The listing builds one solid part. Answer for the finished solid, in the listing's coordinates (mm). Face numbers are marked on the shaded views. A direction names the side the tool comes from. Round coordinates to 2 decimals unless told otherwise and drop trailing zeros. Write each loop counter-clockwise with the first axis right and the second up, starting at its lowest first coordinate (ties: lowest second). Pieces come first, ordered by that corner, then holes. Notation, with made-up numbers: (35, 21.5) - (90, 21.5) arc R14 cw to (90, 44.5) - close; hole circle Ø8 at (-15.5, 87.5). An arc over 180 degrees is marked (long way). Answer in a Markdown table with one row per item.
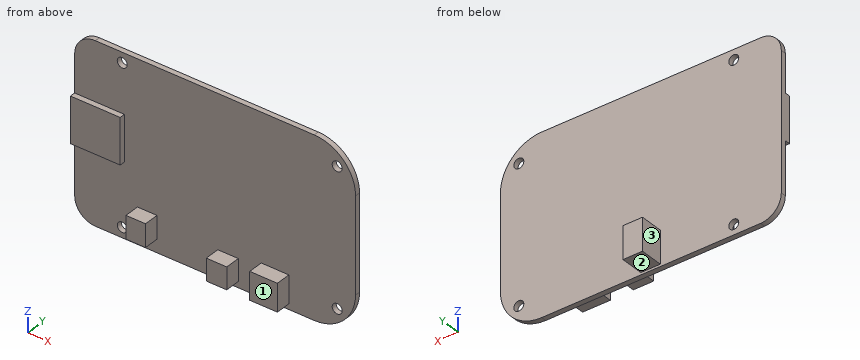
from build123d import *

# Parameters (mm, degrees)
BOSS_EXTRUDE1_DEPTH = 1.6
SKETCH3_R           = 1.53
CUT_EXTRUDE1_DEPTH  = 1.6
SKETCH4_W           = 6
SKETCH4_H           = 10
BOSS_EXTRUDE2_DEPTH = 7.12
SKETCH5_W           = 15.3
SKETCH5_H           = 14
BOSS_EXTRUDE3_DEPTH = 1.7
SKETCH6_W           = 6
SKETCH6_H           = 7
BOSS_EXTRUDE4_DEPTH = 4.6
SKETCH7_W           = 6.3
SKETCH7_H           = 6.75
BOSS_EXTRUDE5_DEPTH = 4.6
SKETCH8_W           = 8.5
SKETCH8_H           = 8.5
BOSS_EXTRUDE6_DEPTH = 4.6


with BuildPart() as part:
    # Sketch1 → Boss-Extrude1 (new body)
    with BuildSketch(Plane(origin=(0, 0, 0), x_dir=(1, 0, 0), z_dir=(0, 1, 0))):
        with BuildLine():
            Line((6.35, 54.61), (73.66, 54.61))
            ThreePointArc((73.66, 54.61), (82.640256121, 50.890256121), (86.36, 41.91))
            Line((86.36, 41.91), (86.36, 12.7))
            ThreePointArc((86.36, 12.7), (82.640256121, 3.719743879), (73.66, 0))
            Line((73.66, 0), (6.35, 0))
            ThreePointArc((6.35, 0), (1.859871939, 1.859871939), (0, 6.35))
            Line((0, 6.35), (0, 48.26))
            ThreePointArc((0, 48.26), (1.859871939, 52.750128061), (6.35, 54.61))
        make_face()
    extrude(amount=BOSS_EXTRUDE1_DEPTH)

    # Sketch3 → Cut-Extrude1 (cut)
    with BuildSketch(Plane(origin=(0, 1.6, 0), x_dir=(1, 0, 0), z_dir=(0, 1, 0))):
        with Locations(Location((80.71, 6.35, 0), (0, 0, 270))):
            Circle(SKETCH3_R)
        with Locations(Location((14.61, 3.11, 0), (0, 0, 270))):
            Circle(SKETCH3_R)
        with Locations(Location((14.61, 51.5, 0), (0, 0, 270))):
            Circle(SKETCH3_R)
        with Locations(Location((80.71, 48.26, 0), (0, 0, 270))):
            Circle(SKETCH3_R)
    extrude(amount=-CUT_EXTRUDE1_DEPTH, mode=Mode.SUBTRACT)

    # Sketch4 → Boss-Extrude2 (add)
    with BuildSketch(Plane(origin=(0, 1.6, 0), x_dir=(1, 0, 0), z_dir=(0, 1, 0))):
        with Locations((40.2, 48.91)):
            Rectangle(SKETCH4_W, SKETCH4_H)
    extrude(amount=BOSS_EXTRUDE2_DEPTH)

    # Sketch5 → Boss-Extrude3 (add)
    with BuildSketch(Plane.XZ):
        with Locations((7.65, -25)):
            Rectangle(SKETCH5_W, SKETCH5_H)
    extrude(amount=BOSS_EXTRUDE3_DEPTH)

    # Sketch6 → Boss-Extrude4 (add)
    with BuildSketch(Plane(origin=(0, 0, 0), x_dir=(-1, 0, 0), z_dir=(0, -1, 0))):
        with Locations((-22.3, 47.11)):
            Rectangle(SKETCH6_W, SKETCH6_H)
    extrude(amount=BOSS_EXTRUDE4_DEPTH)

    # Sketch7 → Boss-Extrude5 (add)
    with BuildSketch(Plane.XZ):
        with Locations((47.15, -49.385)):
            Rectangle(SKETCH7_W, SKETCH7_H)
    extrude(amount=BOSS_EXTRUDE5_DEPTH)

    # Sketch8 → Boss-Extrude6 (add)
    with BuildSketch(Plane.XZ):
        with Locations((61.61, -48.66)):
            Rectangle(SKETCH8_W, SKETCH8_H)
    extrude(amount=BOSS_EXTRUDE6_DEPTH)


solid = part.part
(1) Section A-A (x = 11) is taken. Give the vertices of the cut face in (y, z).
Checked values:
| item | result |
|---|---|
| outline | (-1.7, -32) - (0, -32) - (0, -54.61) - (1.6, -54.61) - (1.6, 0) - (0, 0) - (0, -18) - (-1.7, -18) - close |
(2) Section D-D (x = 80.71) is taken. Give the vertices of the cut face in (y, z), and give its area (3 significant figures).
Checked values:
| item | result |
|---|---|
| outline | (0, -52.47) - (1.6, -52.47) - (1.6, -49.79) - (0, -49.79) - close; (0, -46.73) - (1.6, -46.73) - (1.6, -7.88) - (0, -7.88) - close; (0, -4.82) - (1.6, -4.82) - (1.6, -2.14) - (0, -2.14) - close |
| area | 70.7 mm2 |
(3) Section C-C (y = 5.5) is taken. Give the vertices of the cut face in (x, z).
Checked values:
| item | result |
|---|---|
| outline | (37.2, -53.91) - (43.2, -53.91) - (43.2, -43.91) - (37.2, -43.91) - close |
(4) Find the intervals of material crossed by line 1 (Z direction, x = 80.71, y = 1); line 2 (Y direction, x = 60, z = -30.5); line 3 (X direction, y = 6.25, z = -45.5), in increasing order.
Checked values:
| item | result |
|---|---|
| line 1 | z = -52.47 to -49.79, -46.73 to -7.88, -4.82 to -2.14 |
| line 2 | y = 0 to 1.6 |
| line 3 | x = 37.2 to 43.2 |
(5) Section B-B (z = -3.11) is taken. Give the vertices of the cut face in (x, y).
Checked values:
| item | result |
|---|---|
| outline | (0.89, 0) - (13.08, 0) - (13.08, 1.6) - (0.89, 1.6) - close; (16.14, 0) - (81.99, 0) - (81.99, 1.6) - (16.14, 1.6) - close |
(6) For the marked faces 1, 2 and 3, determine the directions among +Z, -Z, +X, -X, +Y, -Y from which every point of the face is accessible in a straight line to the end or side of a thin tool.
Checked values:
| item | result |
|---|---|
| face 1 | +Z, -Z, +X, -X, -Y |
| face 2 | -Z, +X, -X, +Y |
| face 3 | +Z, -Z, -X, +Y |
(7) Flat-ended cylindrical pins translate along their axes: pin 1 (5 mm diameter, centred on x = 22, z = -13, fed in from +Y); pin 2 (1.4 mm diameter, centred on x = 6, y = -1, fed in from -Z); pin 3 (0.5 mm diameter, centred on x = 5, y = -1.5, fed in from +Z); pin 4 (4 mm diameter, centred on x = 33.5, y = 4.5, fed in from -Z). Find the tip coordinate at first contact, or state that the pin passes through.
Checked values:
| item | result |
|---|---|
| pin 1 | stops at y = 1.6 |
| pin 2 | stops at z = -32 |
| pin 3 | stops at z = -18 |
| pin 4 | passes through |
